Source: CAD feature listing. Evaluate the final solid. Frame: model axes, mm. Face numbers are marked on the shaded views. A direction names the side the tool comes from. Coordinates: 2 decimals unless noted, no trailing zeros. Order: outer loops, then holes, each group sorted by start corner. A loop starts at its lowest first (then second) coordinate and runs counter-clockwise, first axis right, second up. Notation, with made-up numbers: (37, 62) -> (79, 62) arc R12 cw to (79, 79) -> close; hole circle Ø4 at (-4, -16). An arc over 180 degrees is marked (long way). Put each result on its own line as item: value.
from build123d import *

# Parameters (mm, degrees)
F0_R     = 40.346618638
F1_DEPTH = 88.138
F2_SIZE  = 10.16
F3_DEPTH = 88.392
F4_SIZE  = 6.35
F5_DEPTH = 89.916


with BuildPart() as f1:
    # F0 (on Front) → F1 (new body)
    with BuildSketch(Plane.XZ):
        Circle(F0_R)
    extrude(amount=-F1_DEPTH)

    # F2
    f2_edges = [f1.edges().sort_by_distance(p)[0] for p in [
        (-40.346619, 88.138, 0),
    ]]
    chamfer(f2_edges, length=F2_SIZE)

    # F3 (add): a face of the model
    f3_faces = [f1.faces().sort_by_distance(p)[0] for p in [
        (0, 88.138, 0),
    ]]
    extrude(f3_faces, amount=F3_DEPTH)

    # F4
    f4_edges = [f1.edges().sort_by_distance(p)[0] for p in [
        (-30.186619, 176.53, 0),
    ]]
    chamfer(f4_edges, length=F4_SIZE)

    # F5 (add): a face of the model
    f5_faces = [f1.faces().sort_by_distance(p)[0] for p in [
        (0, 176.53, 0),
    ]]
    extrude(f5_faces, amount=F5_DEPTH)


solid = f1.part
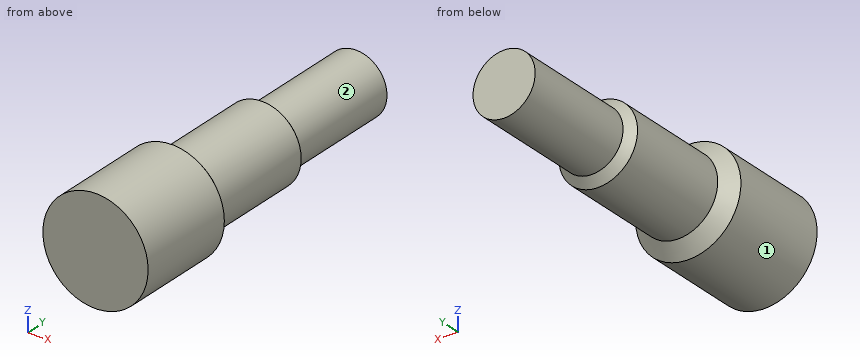
1. Cut plane A-A on z = 0. Output: boundary loops of the cut face in (x, y).
Numbers:
outline: (-40.35, 0) -> (40.35, 0) -> (40.35, 77.98) -> (30.19, 88.14) -> (30.19, 170.18) -> (23.84, 176.53) -> (23.84, 266.45) -> (-23.84, 266.45) -> (-23.84, 176.53) -> (-30.19, 170.18) -> (-30.19, 88.14) -> (-40.35, 77.98) -> close
2. Set-up query: the marked faces 1 and 2. Return all of +Z, -Z, +X, -X, +Y, -Y with unobstructed straight access to the full face (end or side cutting, diameter ignored); none if empty.
Numbers:
face 1: +Y, -Y
face 2: +Y
3. Cut plane C-C on y = 162.5. Output: boundary loops of the cut face in (x, z).
Numbers:
outline: circle Ø60.37 at (0, 0)
4. First-contact query: pin 1 (5 mm diameter, centred on y = 110.5, z = 16.5, fed in from -X); pin 2 (2 mm diameter, centred on y = 235, z = -21.5, fed in from -X); pin 3 (2 mm diameter, centred on y = 184, z = 8, fed in from -X). Flat tips, straight axial feed; report the tip coordinate or a pass-through.
Numbers:
pin 1: stops at x = -26.74
pin 2: stops at x = -12.16
pin 3: stops at x = -22.79
5. Cut plane B-B on x = 0. Output: boundary loops of the cut face in (y, z), plus the area to 3 significant figures.
Numbers:
outline: (0, -40.35) -> (77.98, -40.35) -> (88.14, -30.19) -> (170.18, -30.19) -> (176.53, -23.84) -> (266.45, -23.84) -> (266.45, 23.84) -> (176.53, 23.84) -> (170.18, 30.19) -> (88.14, 30.19) -> (77.98, 40.35) -> (0, 40.35) -> close
area: 16,600 mm2
6. Ray query, line 1 along X through (y, z) = (189, -7); line 2 along X through (y, z) = (98, -1.5); line 3 along Z through (x, y) = (5, 254). Return the intervals inside material, ascending.
Numbers:
line 1: x = -22.79 to 22.79
line 2: x = -30.15 to 30.15
line 3: z = -23.31 to 23.31
